The model under review builds one solid part; all positions refer to its coordinate system, in mm. A direction names the side the tool comes from. Round coordinates to 2 decimals unless told otherwise and drop trailing zeros. Write each loop counter-clockwise with the first axis right and the second up, starting at its lowest first coordinate (ties: lowest second). Pieces come first, ordered by that corner, then holes. Notation, with made-up numbers: (15, 30.5) -> (46, 30.5) arc R4 ccw to (46, 36.5) -> close; hole circle Ø10 at (22, 87.25). An arc over 180 degrees is marked (long way). Return JSON: item names as keys, results as strings. Group by question number.
1. For line 1 along X through (y, z) = (0, -20.5); line 2 along Y through (x, z) = (0, 18); line 3 along Y through (x, z) = (0, 2), list the stretches that pass through material, from the lowest coordinate up. Write a range as from..to.
2. Take a section at D-D, the plane y = -212.5. Write out the cut boundary in (x, z).
3. Clearance check with flat-ended pins moving along their axes: P1, Ø12, axis at x = -152.5, z = 58.5, coming from the -Y side; P2, Ø5, axis at y = 33, z = 54, coming from the +X side; P3, Ø12, axis at x = 216.5, y = -152, coming from the +Z side. State where each tip first meets the part, or that it passes through.
4. Tool access review of faces 1 (the flat face through (-276.5, -3, -22)), 2 (the flat face through (-273.5, -3, -23)), 3 (the cylindrical face through (-10.316, 7.91, -24.65)), 4 (the cylindrical face through (128.982, 118.273, 29.364)), 5 (the cylindrical face through (-237.263, 208.67, 1.479)): name each direction out of +Z, -Z, +X, -X, +Y, -Y from which nothing blocks a thin tool from reaching the whole face with its end or side.
5. Mouldability with a two-part tool opening along Y and no side actions: class faces 6 (the flat face through (-3, 239.5, -23)), 7 (the flat face through (-4, -242.5, -22)), 8 (the flat face through (273.5, -3, -23)) as pulls with the +Y half, pulls with the -Y half, needs draft (parallel to the pull), parting line crosses it, or undercut.
6. Take a section at A-A, the plane z = -27.5. Write out the cut boundary in (x, y).
from build123d import *

# Parameters (mm, degrees)
F2_W     = 553
F2_H     = 485
F2_R     = 10
F2_R_2   = 200
F3_DEPTH = 3
F4_W     = 3
F4_H     = 485
F4_W_2   = 437
F4_H_2   = 3
F5_DEPTH = 50
F6_R     = 13
F6_R_2   = 10
F7_DEPTH = 50


with BuildPart() as f1:
    # F0 (on Front) → F1 (revolve)
    with BuildSketch(Plane.XZ):
        Polygon((-225, 3), (-175, 3), (-175, 55), (-176, 55), (-176, 95), (-224, 95), (-224, 55), (-225, 55), align=None)
        Polygon((-10, 3), (-175, 3), (-225, 3), (-225, 0), (-10, 0), align=None)
    revolve(axis=Axis((0, 0, 187.921241), (0, 0, -1)))

    # F2 (on Top) → F3 (join)
    with BuildSketch(Plane.XY):
        Rectangle(F2_W, F2_H)
        with Locations((-246.5, -212.5)):
            Circle(F2_R, mode=Mode.SUBTRACT)
        with Locations((246.5, -212.5)):
            Circle(F2_R, mode=Mode.SUBTRACT)
        with Locations((-246.5, 212.5)):
            Circle(F2_R, mode=Mode.SUBTRACT)
        Circle(F2_R_2, mode=Mode.SUBTRACT)
        with Locations((246.5, 212.5)):
            Circle(F2_R, mode=Mode.SUBTRACT)
    extrude(amount=F3_DEPTH)

    # F4 (on face) → F5 (join)
    with BuildSketch(Plane.XY.offset(3)):
        with Locations((-275, 0)):
            Rectangle(F4_W, F4_H)
        with Locations((275, 0)):
            Rectangle(F4_W, F4_H)
        with Locations((0, -241)):
            Rectangle(F4_W_2, F4_H_2)
        with Locations((0, 241)):
            Rectangle(F4_W_2, F4_H_2)
    extrude(amount=-F5_DEPTH)

    # F6 (on face) → F7 (join)
    with BuildSketch(Plane(origin=(0, 0, 0), x_dir=(1, 0, 0), z_dir=(0, 0, -1))):
        Circle(F6_R)
        Circle(F6_R_2, mode=Mode.SUBTRACT)
    extrude(amount=F7_DEPTH)


solid = f1.part
Output:
{
 "1": {"line 1": "x = -276.5..-273.5, -13..-10, 10..13, 273.5..276.5", "line 2": "y = -225..-175, 175..225", "line 3": "y = -242.5..-10, 10..242.5"},
 "2": {"outline": "(-276.5, -47) -> (-273.5, -47) -> (-273.5, 0) -> (-256.5, 0) -> (-256.5, 3) -> (-276.5, 3) -> close; (-236.5, 0) -> (236.5, 0) -> (236.5, 3) -> (73.95, 3) -> (73.95, 55) -> (70.85, 55) -> (70.85, 95) -> (-70.85, 95) -> (-70.85, 55) -> (-73.95, 55) -> (-73.95, 3) -> (-236.5, 3) -> close; (256.5, 0) -> (273.5, 0) -> (273.5, -47) -> (276.5, -47) -> (276.5, 3) -> (256.5, 3) -> close"},
 "3": {"P1": "stops at y = -169.8", "P2": "stops at x = 222.92", "P3": "stops at z = 3"},
 "4": {"face 1": "+Z, -Z, -X, +Y, -Y", "face 2": "-Z, +Y, -Y", "face 3": "-Z", "face 4": "+Z", "face 5": "+Z, -Z"},
 "5": {"face 6": "undercut", "face 7": "pulls with the -Y half", "face 8": "needs draft"},
 "6": {"outline": "(-276.5, -242.5) -> (-273.5, -242.5) -> (-273.5, 242.5) -> (-276.5, 242.5) -> close; (-218.5, -242.5) -> (218.5, -242.5) -> (218.5, -239.5) -> (-218.5, -239.5) -> close; (-218.5, 239.5) -> (218.5, 239.5) -> (218.5, 242.5) -> (-218.5, 242.5) -> close; circle Ø26 at (0, 0); (273.5, -242.5) -> (276.5, -242.5) -> (276.5, 242.5) -> (273.5, 242.5) -> close; hole circle Ø20 at (0, 0)"}
}
